CAD build for the part. Positions are in the model's coordinates, mm. Coordinates: 2 decimals unless noted, no trailing zeros. Order: outer loops, then holes, each group sorted by start corner. A loop starts at its lowest first (then second) coordinate and runs counter-clockwise, first axis right, second up. Notation, with made-up numbers: (45, 9.5) - (65, 9.5) arc R30 cw to (65, 39.5) - close; hole circle Ø3 at (30.5, 57.5). An arc over 180 degrees is marked (long way). Write each question's results on one line, items separated by ' | '. Start each with the question number.
Q1. Band-saw the part on C-C, the plane z = 9.5. Write the cut outline in (x, y), then the cut area to 3 significant figures.
Q2. Pull direction Y, two halves, no side cores. Call faces 1 (the cylindrical face through (-0.867, -3.905, 22.605)), 2 (the cylindrical face through (-2.17, -9.76, 14.79)), 3 (the cylindrical face through (1.08, -4.88, 7.4)), 4 (the flat face through (-5, -2, 0)): released by +Y, released by -Y, zero draft, split by the parting line, or undercut.
Q3. Pin check, flat tips, straight feed: P1, Ø8, axis at y = -6.5, z = 4, coming from the -X side; P2, Ø2, axis at x = -1, z = 22.5, coming from the +Y side; P3, Ø6, axis at y = 5.5, z = 23, coming from the +X side; P4, Ø6, axis at y = 5, z = 22, coming from the -X side. Stop position of each tip, or through.
Q4. Band-saw the part on D-D, the plane x = 4.5. Write the cut outline in (y, z).
Q5. Wall check: probe 1 along Y at (x, z) = (0, 18.75); probe 2 along Y at (x, z) = (0, 6.5); probe 3 along X at (y, z) = (-2.5, 26). Give the ranges that are in metal, low to high.
Q6. Band-saw the part on A-A, the plane y = 0. Write the cut outline in (x, z), then the cut area to 3 significant figures.
```python
from build123d import *

# Parameters (mm, degrees)
SKETCH1_R           = 10
SKETCH1_R_2         = 0.065570397
BOSS_EXTRUDE1_DEPTH = 30
SKETCH2_R           = 4
CUT_EXTRUDE1_DEPTH  = 30
SKETCH3_R           = 5
CUT_EXTRUDE2_DEPTH  = 15


with BuildPart() as part:
    # Sketch1 → Boss-Extrude1 (new body)
    with BuildSketch(Plane.XY):
        Circle(SKETCH1_R)
        Circle(SKETCH1_R_2, mode=Mode.SUBTRACT)
    extrude(amount=BOSS_EXTRUDE1_DEPTH)

    # Sketch2 → Cut-Extrude1 (cut)
    with BuildSketch(Plane.XY.offset(30)):
        Circle(SKETCH2_R)
    extrude(amount=-CUT_EXTRUDE1_DEPTH, mode=Mode.SUBTRACT)

    # Sketch3 → Cut-Extrude2 (cut)
    with BuildSketch(Plane(origin=(0, 0, 0), x_dir=(-1, 0, 0), z_dir=(0, 0, -1))):
        Circle(SKETCH3_R)
    extrude(amount=-CUT_EXTRUDE2_DEPTH, mode=Mode.SUBTRACT)


solid = part.part
```
Results below:
1) outline: circle Ø20 at (0, 0); hole circle Ø10 at (0, 0) | area: 236 mm²
2) face 1: undercut | face 2: split by the parting line | face 3: undercut | face 4: zero draft
3) P1: stops at x = -9.68 | P2: stops at y = 10 | P3: stops at x = 9.68 | P4: stops at x = -9.8
4) outline: (-8.93, 0) - (-2.18, 0) - (-2.18, 15) - (2.18, 15) - (2.18, 0) - (8.93, 0) - (8.93, 30) - (-8.93, 30) - close
5) probe 1: y = -10 to -4, 4 to 10 | probe 2: y = -10 to -5, 5 to 10 | probe 3: x = -9.68 to -3.12, 3.12 to 9.68
6) outline: (-10, 0) - (-5, 0) - (-5, 15) - (-4, 15) - (-4, 30) - (-10, 30) - close; (4, 15) - (5, 15) - (5, 0) - (10, 0) - (10, 30) - (4, 30) - close | area: 330 mm²
